For this review, take the finished solid that the model builds, in its own axes (mm). Face numbers are marked on the shaded views. A direction names the side the tool comes from. Coordinates: 2 decimals unless noted, no trailing zeros. Write each loop counter-clockwise with the first axis right and the second up, starting at its lowest first coordinate (ties: lowest second). Pieces come first, ordered by that corner, then holes.
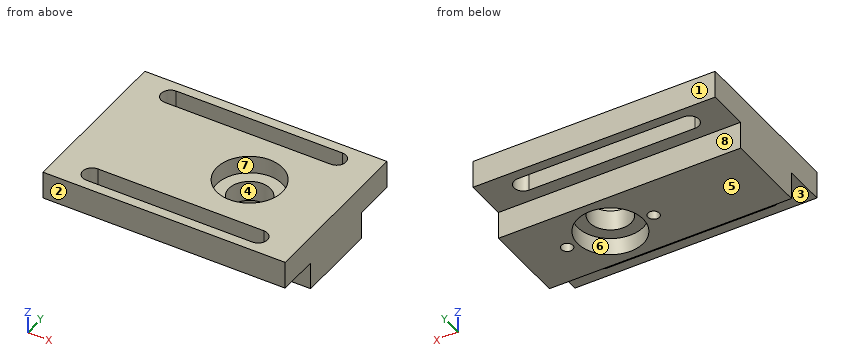
```python
from build123d import *

# Parameters (mm, degrees)
SKETCH_1_W             = 70
SKETCH_1_H             = 48
EXTRUDE_1_DEPTH        = 8
SKETCH_2_W             = 70
SKETCH_2_H             = 24
EXTRUDE_2_DEPTH        = 8
SKETCH_3_R             = 6
CUT_EXTRUDE_1_DEPTH    = 87.371291527
SKETCH_6_R             = 9.5
CUT_EXTRUDE_4_DEPTH    = 5
CUT_EXTRUDE_START      = -5.1
SKETCH_7_R             = 9.5
CUT_EXTRUDE_5_DEPTH    = 5.1
HOLE_WIZARD_M4_1_D     = 3.3
HOLE_WIZARD_M4_1_DEPTH = 10.1
HOLE_WIZARD_M4_1_TIP   = 0.991420021
CUT_EXTRUDE_6_DEPTH    = 87.371291527


with BuildPart() as part:
    # 草图1 → 凸台-拉伸1 (new body)
    with BuildSketch(Plane.XY):
        with Locations((35, 24)):
            Rectangle(SKETCH_1_W, SKETCH_1_H)
    extrude(amount=EXTRUDE_1_DEPTH)

    # 草图2 → 凸台-拉伸2 (add)
    with BuildSketch(Plane(origin=(0, 0, 0), x_dir=(-1, 0, 0), z_dir=(0, 0, -1))):
        with Locations((-35, 24)):
            Rectangle(SKETCH_2_W, SKETCH_2_H)
    extrude(amount=EXTRUDE_2_DEPTH)

    # 草图3 → 切除-拉伸1 (cut, through all)
    with BuildSketch(Plane(origin=(0, 0, -8), x_dir=(-1, 0, 0), z_dir=(0, 0, -1))):
        with Locations((-45, 24)):
            Circle(SKETCH_3_R)
    extrude(amount=-CUT_EXTRUDE_1_DEPTH, mode=Mode.SUBTRACT)

    # 草图6 → 切除-拉伸4 (cut)
    with BuildSketch(Plane(origin=(0, 0, -8), x_dir=(-1, 0, 0), z_dir=(0, 0, -1))):
        with Locations((-45, 24)):
            Circle(SKETCH_6_R)
    extrude(amount=-CUT_EXTRUDE_4_DEPTH, mode=Mode.SUBTRACT)

    # 草图7 → 切除-拉伸5 (cut)
    with BuildSketch(Plane.XY.offset(8).offset(CUT_EXTRUDE_START)):
        with Locations(Location((45, 24, 0), (0, 0, 180))):
            Circle(SKETCH_7_R)
    extrude(amount=CUT_EXTRUDE_5_DEPTH, mode=Mode.SUBTRACT)

    # M4 螺纹孔1
    with Locations(Plane(origin=(0, 0, -8), x_dir=(-1, 0, 0), z_dir=(0, 0, -1))):
        with Locations((-57.5, 24), (-32.5, 24)):
            Hole(HOLE_WIZARD_M4_1_D / 2, depth=HOLE_WIZARD_M4_1_DEPTH)
            with Locations((0, 0, -(HOLE_WIZARD_M4_1_DEPTH + HOLE_WIZARD_M4_1_TIP / 2))):  # 118° drill point
                Cone(0, HOLE_WIZARD_M4_1_D / 2, HOLE_WIZARD_M4_1_TIP, mode=Mode.SUBTRACT)

    # 草图10 → 切除-拉伸6 (cut, through all)
    with BuildSketch(Plane.XY.offset(8)):
        with BuildLine():
            Line((10.800456012, 45.2), (58.800456012, 45.2))
            ThreePointArc((58.800456012, 45.2), (61.500456012, 42.5), (58.800456012, 39.8))
            Line((58.800456012, 39.8), (10.800456012, 39.8))
            ThreePointArc((10.800456012, 39.8), (8.100456012, 42.5), (10.800456012, 45.2))
        make_face()
        with BuildLine():
            Line((10.800456012, 2.8), (58.800456012, 2.8))
            ThreePointArc((58.800456012, 2.8), (61.500456012, 5.5), (58.800456012, 8.2))
            Line((58.800456012, 8.2), (10.800456012, 8.2))
            ThreePointArc((10.800456012, 8.2), (8.100456012, 5.5), (10.800456012, 2.8))
        make_face()
    extrude(amount=-CUT_EXTRUDE_6_DEPTH, mode=Mode.SUBTRACT)


solid = part.part
```
Q1. Add section A-A (x = 14). State the section outline as (y, z) points.
Ans:
outline: (0, 0) - (2.8, 0) - (2.8, 8) - (0, 8) - close; (8.2, 0) - (12, 0) - (12, -8) - (36, -8) - (36, 0) - (39.8, 0) - (39.8, 8) - (8.2, 8) - close; (45.2, 0) - (48, 0) - (48, 8) - (45.2, 8) - close
Q2. Tool access review of the marked faces 5, 6, 7 and 8: name each direction out of +Z, -Z, +X, -X, +Y, -Y from which nothing blocks a thin tool from reaching the whole face with its end or side.
Ans:
face 5: -Z, +X, -X, +Y, -Y
face 6: -Z
face 7: +Z
face 8: -Z, +X, -X, +Y
Q3. Add section B-B (z = 4.75). State the section outline as (x, y) points.
Ans:
outline: (0, 0) - (70, 0) - (70, 48) - (0, 48) - close; hole (10.8, 2.8) - (58.8, 2.8) arc R2.7 ccw to (58.8, 8.2) - (10.8, 8.2) arc R2.7 ccw to start; hole (10.8, 39.8) - (58.8, 39.8) arc R2.7 ccw to (58.8, 45.2) - (10.8, 45.2) arc R2.7 ccw to start; hole circle Ø19 at (45, 24)
Q4. Draft analysis for pull direction Y (two halves, no side actions). For the marked faces 1, 2, 3 and 4, state which applies: +Y half, -Y half, draft (parallel to the pull), parting line (faces both ways), or undercut.
Ans:
face 1: +Y half
face 2: -Y half
face 3: draft
face 4: undercut
Q5. For probe 1 along Y at (x, z) = (45, 6.45); probe 2 along Y at (x, z) = (13, 3.25); probe 3 along Y at (x, z) = (45, 0.45), list the stretches that pass through material, from the lowest coordinate up.
Ans:
probe 1: y = 0 to 2.8, 8.2 to 14.5, 33.5 to 39.8, 45.2 to 48
probe 2: y = 0 to 2.8, 8.2 to 39.8, 45.2 to 48
probe 3: y = 0 to 2.8, 8.2 to 18, 30 to 39.8, 45.2 to 48
Q6. Add section C-C (y = 42.5). State the section outline as (x, z) points, then the cut area to 3 significant figures.
Ans:
outline: (0, 0) - (8.1, 0) - (8.1, 8) - (0, 8) - close; (61.5, 0) - (70, 0) - (70, 8) - (61.5, 8) - close
area: 133 mm2
Q7. Clearance check with flat-ended pins moving along their axes: pin 1 Ø11.5 at (x, y) = (45, 24) entering from -Z; pin 2 Ø9.5 at (x, y) = (27, 44) entering from -Z; pin 3 Ø6.5 at (x, z) = (28, -4) entering from +Y. State where each tip first meets the part, or that it passes through.
Ans:
pin 1: passes through
pin 2: stops at z = 0
pin 3: stops at y = 36
Q8. Add section D-D (z = 1). State the section outline as (x, y) points, then the cut area to 3 significant figures.
Ans:
outline: (0, 0) - (70, 0) - (70, 48) - (0, 48) - close; hole (10.8, 2.8) - (58.8, 2.8) arc R2.7 ccw to (58.8, 8.2) - (10.8, 8.2) arc R2.7 ccw to start; hole (10.8, 39.8) - (58.8, 39.8) arc R2.7 ccw to (58.8, 45.2) - (10.8, 45.2) arc R2.7 ccw to start; hole circle Ø3.3 at (32.5, 24); hole circle Ø12 at (45, 24); hole circle Ø3.3 at (57.5, 24)
area: 2,670 mm2
